Could you check a few things on this drawing? It's one solid part, dimensions in mm from its lowest x, y, z. Give positions to 0.01 mm unless a question says otherwise; leave off trailing zeros. Write each loop counter-clockwise with the first axis right and the second up, starting at its lowest first coordinate (ties: lowest second). Pieces come first, ordered by that corner, then holes. Notation, with made-up numbers: (17.5, 38) - (36.5, 38) arc R12 ccw to (36.5, 48) - close; hole circle Ø11 at (5, 80). An arc over 180 degrees is marked (long way). One line per item, written item: value. Start each with the question number.
1) Imagine slicing it at B-B on x = 145. Write out the boundary of the cut face in (y, z), plus the area to 3 significant figures.
2) I'm going to push flat-ended pins straight in: P1, Ø2, axis at x = 139, y = 170, coming from the -Z side; P2, Ø3, axis at x = 154, z = 3.5, coming from the +Y side; P3, Ø16, axis at x = 145, y = 316, coming from the +Z side. Where does each tip first touch, or does it pass through?
3) Imagine slicing it at C-C on z = 4.35. Write out the boundary of the cut face in (x, y).
4) Imagine slicing it at D-D on y = 101. Write out the boundary of the cut face in (x, z).
5) Imagine slicing it at A-A on y = 256. Write out the boundary of the cut face in (x, z), plus the area to 3 significant figures.
6) Please list where these lines run through material, in increasing order: L1, parallel to X at y = 316, z = 1.75; L2, parallel to Y at x = 145, z = 4.75; L3, parallel to Y at x = 145.5, z = 4.35. Write a range as [from, to].
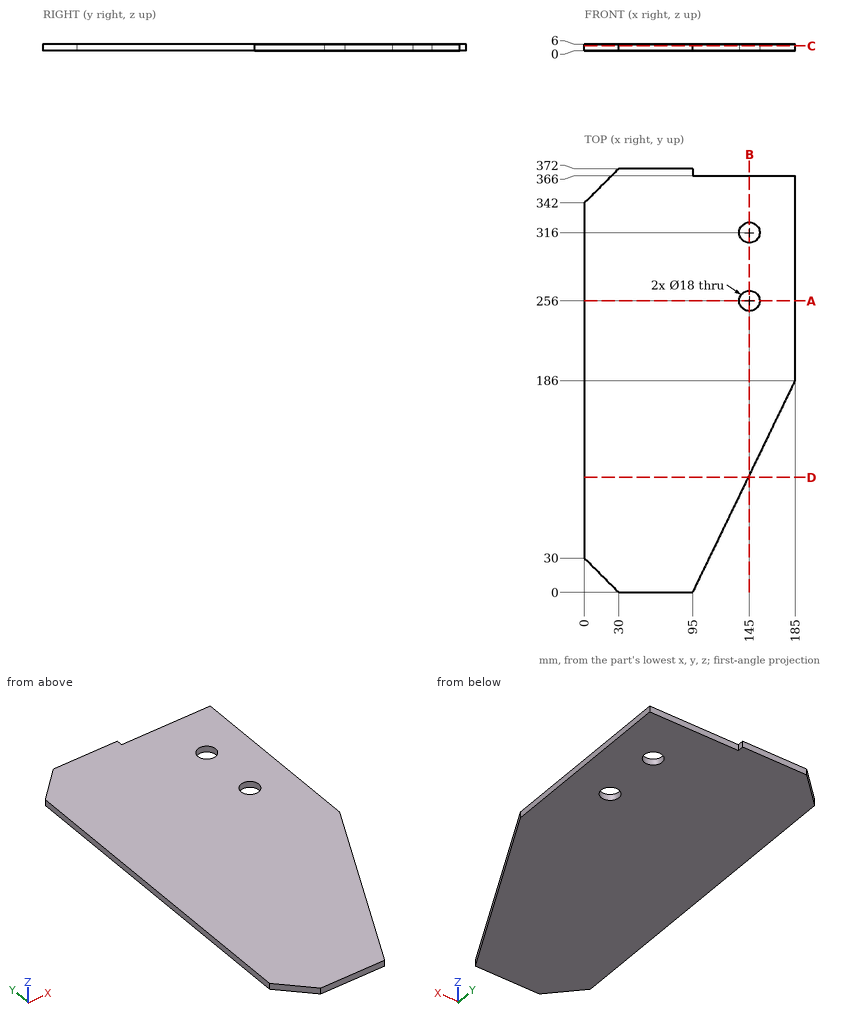
Numbers:
1. outline: (103.33, 0) - (247, 0) - (247, 6) - (103.33, 6) - close; (265, 0) - (307, 0) - (307, 6) - (265, 6) - close; (325, 0) - (366, 0) - (366, 6) - (325, 6) - close
1. area: 1,360 mm^2
2. P1: z = 0
2. P2: y = 366
2. P3: through
3. outline: (0, 30) - (30, 0) - (95, 0) - (185, 186) - (185, 366) - (95, 366) - (95, 372) - (30, 372) - (0, 342) - close; hole circle Ø18 at (145, 256); hole circle Ø18 at (145, 316)
4. outline: (0, 0) - (143.87, 0) - (143.87, 6) - (0, 6) - close
5. outline: (0, 0) - (136, 0) - (136, 6) - (0, 6) - close; (154, 0) - (185, 0) - (185, 6) - (154, 6) - close
5. area: 1,000 mm^2
6. L1: [0, 136], [154, 185]
6. L2: [103.33, 247], [265, 307], [325, 366]
6. L3: [104.37, 247.01], [264.99, 307.01], [324.99, 366]
